Part model, mm, in its own coordinate system. Face numbers are marked on the shaded views. A direction names the side the tool comes from. Give positions to 0.01 mm unless a question says otherwise; leave off trailing zeros. Order: outer loops, then holes, each group sorted by start corner. A loop starts at its lowest first (then second) coordinate and runs counter-clockwise, first axis right, second up. Notation, with made-up numbers: (86.25, 14.25) - (91.25, 14.25) arc R35 cw to (91.25, 50.25) - close; hole circle Ø11 at (20, 7.5). An arc over 180 degrees is marked (long way). One line per item, written item: value.
```python
from build123d import *

# Parameters (mm, degrees)
SKETCH1_R                                        = 20
EXTRUDE1_DEPTH                                   = 3
SKETCH2_R                                        = 9
EXTRUDE2_DEPTH                                   = 6
SKETCH3_R                                        = 9
EXTRUDE3_DEPTH                                   = 33
CUT_SWEEP1_PITCH                                 = 10
SKETCH6_R                                        = 4
EXTRUDE4_DEPTH                                   = 9
CBORE_FOR_M3_PAN_HEAD_MACHINE_SCREW1_D           = 3
CBORE_FOR_M3_PAN_HEAD_MACHINE_SCREW1_CBORE_D     = 6.5
CBORE_FOR_M3_PAN_HEAD_MACHINE_SCREW1_CBORE_DEPTH = 2
SKETCH8_R                                        = 2
EXTRUDE5_DEPTH                                   = 59.318093247
SKETCH9_R                                        = 3.25
EXTRUDE6_DEPTH                                   = 3


with BuildPart() as part:
    # Sketch1 → Extrude1 (new body)
    with BuildSketch(Plane.XY):
        Circle(SKETCH1_R)
    extrude(amount=EXTRUDE1_DEPTH)

    # Sketch2 → Extrude2 (add)
    with BuildSketch(Plane.XY.offset(3)):
        Circle(SKETCH2_R)
    extrude(amount=EXTRUDE2_DEPTH)

    # Sketch3 → Extrude3 (add)
    with BuildSketch(Plane.XY.offset(9)):
        Circle(SKETCH3_R)
    extrude(amount=EXTRUDE3_DEPTH)

    # Cut-Sweep1: arcs per turn and ends read off the stored shape
    # Cut-Sweep1: the profile of Sketch5 screwed along a right-hand helix through 4 turns, 8 arcs to a turn; built about Z, then put on its axis
    cut_sweep1_z = Axis((0, 0, 0), (0, 0, 1))
    cut_sweep1_corners = [(5.437822174, 0, -8.556624327), (5.437822174, 0, -11.443375673), (12.031088913, 0, -15.25), (12.031088913, 0, -4.75)]
    with BuildLine(mode=Mode.PRIVATE) as cut_sweep1_profile:
        Line(cut_sweep1_corners[0], cut_sweep1_corners[1])
        Line(cut_sweep1_corners[1], cut_sweep1_corners[2])
        Line(cut_sweep1_corners[2], cut_sweep1_corners[3])
        Line(cut_sweep1_corners[3], cut_sweep1_corners[0])
    cut_sweep1_cap = Face(cut_sweep1_profile.wire())
    cut_sweep1_turn_angles = [0, 22.5, 45, 67.5, 90, 112.5, 135, 157.5, 180, 202.5, 225, 247.5, 270, 292.5, 315, 337.5, 360]
    cut_sweep1_turn_weights = [1, 0.9238795325112867, 1, 0.9238795325112867, 1, 0.9238795325112867, 1, 0.9238795325112867, 1, 0.9238795325112867, 1, 0.9238795325112867, 1, 0.9238795325112867, 1, 0.9238795325112867, 1]
    cut_sweep1_turn_rails = [Edge.make_bspline([Vector(p[0], p[1], 0).rotate(cut_sweep1_z, cut_sweep1_turn_angles[k]) / cut_sweep1_turn_weights[k] + Vector(0, 0, p[2] + CUT_SWEEP1_PITCH * cut_sweep1_turn_angles[k] / 360) for k in range(17)], [0, 0, 0, 1, 1, 2, 2, 3, 3, 4, 4, 5, 5, 6, 6, 7, 7, 8, 8, 8], 2, cut_sweep1_turn_weights) for p in cut_sweep1_corners]
    cut_sweep1_turn_sides = [Face.make_surface_from_curves(cut_sweep1_turn_rails[p[0]], cut_sweep1_turn_rails[p[1]]) for p in [(0, 1), (1, 2), (2, 3), (3, 0)]]
    cut_sweep1 = Plane(origin=(0, 0, 42), x_dir=(-1, 0, 0), z_dir=(0, 0, -1)) * Solid(Shell([*[p.moved(Location((0, 0, CUT_SWEEP1_PITCH * i))) for i in range(4) for p in cut_sweep1_turn_sides], cut_sweep1_cap, cut_sweep1_cap.rotate(cut_sweep1_z, 1440).moved(Location((0, 0, CUT_SWEEP1_PITCH * 1440 / 360)))]))
    add(cut_sweep1, mode=Mode.SUBTRACT)

    # Sketch6 → Extrude4 (add)
    with BuildSketch(Plane.XY.offset(42)):
        Circle(SKETCH6_R)
    extrude(amount=EXTRUDE4_DEPTH)

    # CBORE for M3 Pan Head Machine Screw1 (through all)
    with Locations(Plane(origin=(15, 0, 3), x_dir=(1, 0, 0), z_dir=(0, 0, 1))):
        with Locations((0, 0), (-15, -15), (-30, 0), (-15, 15)):
            CounterBoreHole(CBORE_FOR_M3_PAN_HEAD_MACHINE_SCREW1_D / 2, CBORE_FOR_M3_PAN_HEAD_MACHINE_SCREW1_CBORE_D / 2, CBORE_FOR_M3_PAN_HEAD_MACHINE_SCREW1_CBORE_DEPTH)

    # Sketch8 → Extrude5 (cut, through all)
    with BuildSketch(Plane(origin=(0, 0, 0), x_dir=(-1, 0, 0), z_dir=(0, 0, -1))):
        Circle(SKETCH8_R)
    extrude(amount=-EXTRUDE5_DEPTH, mode=Mode.SUBTRACT)

    # Sketch9 → Extrude6 (cut)
    with BuildSketch(Plane(origin=(0, 0, 0), x_dir=(-1, 0, 0), z_dir=(0, 0, -1))):
        Circle(SKETCH9_R)
    extrude(amount=-EXTRUDE6_DEPTH, mode=Mode.SUBTRACT)


solid = part.part
```
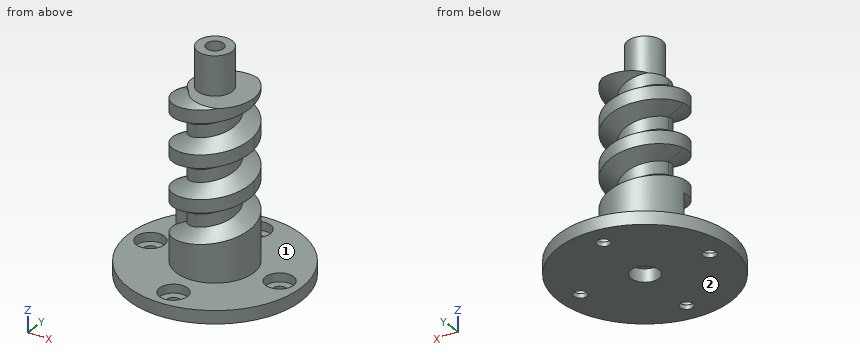
1) Slice it at A-A on x = 15.5. Write the cut outline in (y, z), then the cut area to 3 significant figures.
Answer:
outline: (-12.64, 0) - (-1.41, 0) - (-1.41, 1) - (-3.21, 1) - (-3.21, 3) - (-12.64, 3) - close; (1.41, 0) - (12.64, 0) - (12.64, 3) - (3.21, 3) - (3.21, 1) - (1.41, 1) - close
area: 60.2 mm2
2) Wall check: line 1 along Y through (x, z) = (0, 2.05); line 2 along Z through (x, y) = (-2, 12.5); line 3 along Y through (x, z) = (-15, 2.4). Give the ranges that are in metal, low to high. Write a range as [from, to].
Answer:
line 1: y = [-20, -18.25], [-11.75, -3.25], [3.25, 11.75], [18.25, 20]
line 2: z = [0, 1]
line 3: y = [-13.23, -3.25], [3.25, 13.23]
3) Slice it at D-D on x = 0. Count the separate pieces of the cut face and the enclosed holes in it, then the cut area to 3 significant figures.
Answer:
separate pieces: 4
enclosed holes: 0
area: 545 mm2
4) Slice it at B-B on y = 15. Write the cut outline in (x, z), then the cut area to 3 significant figures.
Answer:
outline: (-13.23, 0) - (-1.5, 0) - (-1.5, 1) - (-3.25, 1) - (-3.25, 3) - (-13.23, 3) - close; (1.5, 0) - (13.23, 0) - (13.23, 3) - (3.25, 3) - (3.25, 1) - (1.5, 1) - close
area: 63.4 mm2
5) Which spindle directions (+Z, -Z, +X, -X, +Y, -Y) get a long thin tool onto all of the face, cutting with end or side? Do the marked faces 1 and 2. Say none if no direction does.
Answer:
face 1: +Z
face 2: -Z, +X, -X, +Y, -Y
6) Drop flat-ended pins along their axis: P1, Ø5, axis at x = -6.5, z = 20.5, coming from the -Y side; P2, Ø4.5, axis at x = 0, y = 0, coming from the -Z side; P3, Ø10, axis at y = 6, z = 22.5, coming from the -X side. Give the stop position or say it passes through.
Answer:
P1: stops at y = -8.06
P2: stops at z = 3
P3: stops at x = -8.82
7) Slice it at C-C on z = 44.5. Write the cut outline in (x, y).
Answer:
outline: circle Ø8 at (0, 0); hole circle Ø4 at (0, 0)
